Part model, mm, in its own coordinate system. Face numbers are marked on the shaded views. A direction names the side the tool comes from. Round coordinates to 2 decimals unless told otherwise and drop trailing zeros. Order: outer loops, then holes, each group sorted by start corner. A loop starts at its lowest first (then second) coordinate and runs counter-clockwise, first axis right, second up. Notation, with made-up numbers: (-2, 9) -> (13, 9) arc R36 ccw to (13, 45) -> close; hole circle Ø11 at (-38, -5). An arc over 180 degrees is marked (long way). Return JSON: item names as keys, results as strings. Group by question number.
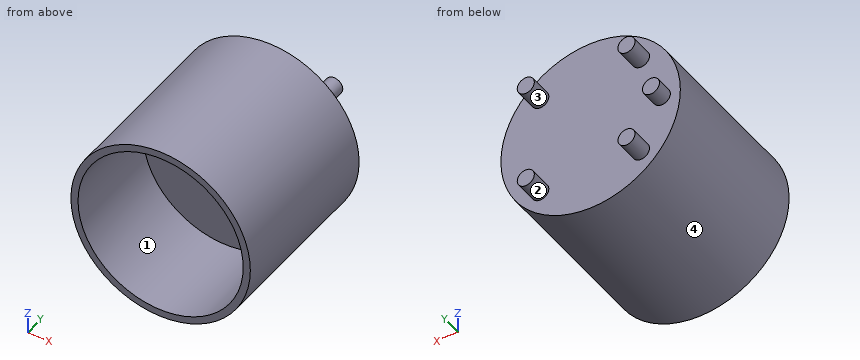
Autodesk Inventor part; units mm, degrees
ref_plane "YZ Plane" through (0, 0, 0) normal (1, 0, 0) x (0, 1, 0)
ref_plane "XZ Plane" through (0, 0, 0) normal (0, 1, 0) x (-1, 0, 0)
ref_plane "XY Plane" through (0, 0, 0) normal (0, 0, 1) x (1, 0, 0)
sketch "Sketch4" plane through (0, 0, 0) normal (0, 1, 0) x (-1, 0, 0)
  circle A0 centre (0, 0) radius 31.5
  dimension "d7" = 63
extrude "Extrusion4" add sketch "Sketch4" along normal blind 60
sketch "Sketch6" plane through (0, 60, 0) normal (0, 1, 0) x (1, 0, 0)
  circle A0 centre (0, 0) radius 25
  circle A1 centre (-25, 0) radius 3
  dimension "d22" = 50
  dimension "d23" = 6
extrude "Extrusion6" add sketch "Sketch6" along normal blind 6 contours A1 A0 | A0 A1 picked at (-23.9867, 0) picked at (-25.9867, 0)
sketch "Sketch7" plane through (0, 60, 0) normal (0, 1, 0) x (1, 0, 0)
  line L0 (0, 0) -> (21.0028, 0) construction
  line L1 (0, 0) -> (25, 0) construction
  line L2 (0, 0) -> (25, 0) construction
  circle A0 centre (-17.6777, -17.6777) radius 3
  circle A1 centre (-17.6777, 17.6777) radius 3
  circle A2 centre (17.6777, 17.6777) radius 3
  circle A3 centre (17.6777, -17.6777) radius 3
  dimension "d34" = 6
  dimension "d35" = 6
  dimension "d36" = 6
  dimension "d37" = 6
extrude "Extrusion7" add sketch "Sketch7" along normal blind 8
thread "Thread1"
thread "Thread2"
thread "Thread3"
thread "Thread4"
sketch "Sketch8" plane through (0, 0, 0) normal (0, -1, 0) x (1, 0, 0)
  circle A0 centre (0, 0) radius 29
extrude "Extrusion8" cut sketch "Sketch8" against normal blind 36
thread "Thread5"
sketch "Sketch9" plane through (0, 36, 0) normal (0, -1, 0) x (1, 0, 0)
  point P0 (0, 0)
thread "Thread6"
properties part number "platform"
(1) Pin check, flat tips, straight feed: P1, Ø1.5, axis at x = 17.5, y = 14.5, coming from the -Z side; P2, Ø12, axis at y = 7, z = -24.5, coming from the +X side; P3, Ø6.5, axis at x = -23.5, z = -1, coming from the +Y side. Stop position of each tip, or through.
(2) Tool access for the marked faces 1 and 2: list every direction of +Z, -Z, +X, -X, +Y, -Y with a clear straight run to the whole face (end or side of a thin tool).
(3) Saw through at D-D, the plane y = 43.5. List the corners of the cut face in (x, z).
(4) Saw through at B-B, the plane y = 5. List the corners of the cut face in (x, z), and give its area (3 significant figures).
(5) Probe L1, parallel to Z at x = 0, y = 18; L2, parallel to Y at x = 19.5, z = -24.5; L3, parallel to Y at x = 23, z = 0.5. List the from-to ranges inside material, lowest first. Write a range as [from, to].
(6) Saw through at C-C, the plane z = 0. List the corners of the cut face in (x, y).
(7) Saw through at A-A, the plane x = 0. List the corners of the cut face in (y, z).
(8) Mould opens along Z. For the marked faces 3 and 4 say: pulls with the +Z half, pulls with the -Z half, needs draft (parallel to the pull), parting line crosses it, or undercut.
Results are:
{
 "1": {"P1": "stops at z = -26.68", "P2": "stops at x = 25.5", "P3": "stops at y = 66"},
 "2": {"face 1": "-Y", "face 2": "+Y"},
 "3": {"outline": "circle Ø63 at (0, 0)"},
 "4": {"outline": "circle Ø63 at (0, 0); hole circle Ø58 at (0, 0)", "area": "475 mm^2"},
 "5": {"L1": "z = [-31.5, -29], [29, 31.5]", "L2": "y = [0, 60]", "L3": "y = [36, 60]"},
 "6": {"outline": "(-31.5, 0) -> (-29, 0) -> (-29, 36) -> (29, 36) -> (29, 0) -> (31.5, 0) -> (31.5, 60) -> (-22, 60) -> (-22, 66) -> (-28, 66) -> (-28, 60) -> (-31.5, 60) -> close"},
 "7": {"outline": "(0, -31.5) -> (60, -31.5) -> (60, 31.5) -> (0, 31.5) -> (0, 29) -> (36, 29) -> (36, -29) -> (0, -29) -> close"},
 "8": {"face 3": "undercut", "face 4": "parting line crosses it"}
}
